Build history of the part. All positions in model axes, mm. Face numbers are marked on the shaded views. A direction names the side the tool comes from. Give positions to 0.01 mm unless a question says otherwise; leave off trailing zeros. Order: outer loops, then holes, each group sorted by start corner. A loop starts at its lowest first (then second) coordinate and runs counter-clockwise, first axis right, second up. Notation, with made-up numbers: (-14.5, 17.25) -> (34.5, 17.25) arc R10 ccw to (34.5, 28.25) -> close; hole circle Ø5 at (63, -24). An arc over 180 degrees is marked (long way). Write item = value, one per line. Start each with the question number.
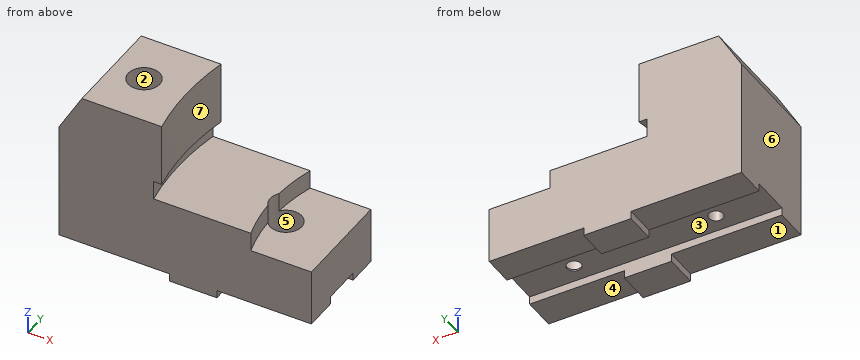
from build123d import *

# Parameters (mm, degrees)
SKETCH_W        = 160
SKETCH_H        = 65
PAD_DEPTH       = 100
POCKET_DEPTH    = 65.001
SKETCH002_R     = 4.5
POCKET001_DEPTH = 100.001
SKETCH003_R     = 10
POCKET002_DEPTH = 30
SKETCH004_R     = 170
POCKET003_DEPTH = 40
SKETCH005_R     = 175
POCKET004_DEPTH = 12
SKETCH006_R     = 115
POCKET005_DEPTH = 12
SKETCH007_R     = 4.5
POCKET006_DEPTH = 36.001
SKETCH008_R     = 10
POCKET009_DEPTH = 30
SKETCH009_W     = 30
SKETCH009_H     = 14.232688
PAD001_DEPTH    = 65
SKETCH010_W     = 25
SKETCH010_H     = 15.667085
POCKET010_DEPTH = 160.001


with BuildPart() as part:
    # Sketch → Pad (new body)
    with BuildSketch(Plane.XY):
        Rectangle(SKETCH_W, SKETCH_H)
    extrude(amount=PAD_DEPTH)

    # Sketch001 → Pocket (cut, through all)
    with BuildSketch(Plane.XZ.offset(32.5)):
        Polygon((-80, 100), (-80, 75), (-65.566243, 100), align=None)
    extrude(amount=-POCKET_DEPTH, mode=Mode.SUBTRACT)

    # Sketch002 → Pocket001 (cut, through all)
    with BuildSketch(Plane.XY.offset(100)):
        with Locations((-45, 0)):
            Circle(SKETCH002_R)
    extrude(amount=-POCKET001_DEPTH, mode=Mode.SUBTRACT)

    # Sketch003 → Pocket002 (cut)
    with BuildSketch(Plane.XY.offset(100)):
        with Locations((-45, 0)):
            Circle(SKETCH003_R)
    extrude(amount=-POCKET002_DEPTH, mode=Mode.SUBTRACT)

    # Sketch004 → Pocket003 (cut)
    with BuildSketch(Plane.XY.offset(100)):
        with Locations((151.864466, 0)):
            Circle(SKETCH004_R)
    extrude(amount=-POCKET003_DEPTH, mode=Mode.SUBTRACT)

    # Sketch005 → Pocket004 (cut)
    with BuildSketch(Plane.XY.offset(60)):
        with Locations((151.864466, 0)):
            Circle(SKETCH005_R)
    extrude(amount=-POCKET004_DEPTH, mode=Mode.SUBTRACT)

    # Sketch006 → Pocket005 (cut)
    with BuildSketch(Plane.XY.offset(48)):
        with Locations((151.864466, 0)):
            Circle(SKETCH006_R)
    extrude(amount=-POCKET005_DEPTH, mode=Mode.SUBTRACT)

    # Sketch007 → Pocket006 (cut, through all)
    with BuildSketch(Plane.XY.offset(36)):
        with Locations((45, 0)):
            Circle(SKETCH007_R)
    extrude(amount=-POCKET006_DEPTH, mode=Mode.SUBTRACT)

    # Sketch008 → Pocket009 (cut, symmetric)
    with BuildSketch(Plane.XY.offset(36)):
        with Locations((45, 0)):
            Circle(SKETCH008_R)
    extrude(amount=POCKET009_DEPTH, both=True, mode=Mode.SUBTRACT)

    # Sketch009 → Pad001 (new body)
    with BuildSketch(Plane.XZ.offset(32.5)):
        with Locations((5, 2.116344)):
            Rectangle(SKETCH009_W, SKETCH009_H)
    extrude(amount=-PAD001_DEPTH)

    # Sketch010 → Pocket010 (cut, through all)
    with BuildSketch(Plane.YZ.offset(80)):
        with Locations((0.638302, -2.833543)):
            Rectangle(SKETCH010_W, SKETCH010_H)
    extrude(amount=-POCKET010_DEPTH, mode=Mode.SUBTRACT)


solid = part.part
(1) Mould opens along X. For the marked faces 4, 5, 6 and 7 say: released by +X, released by -X, zero draft, split by the parting line, or undercut.
(2) Cut at C-C, the plane z = 16.5. Give the cut face in (x, y).
(3) Flat gauge pins, fed straight in: P1, Ø5.5, axis at y = 23, z = -3.5, coming from the -X side; P2, Ø10.5, axis at x = -49, y = -17.5, coming from the -Z side; P3, Ø10.5, axis at x = 45, y = 0, coming from the -Z side. Where does each tip first touch, or does it go through?
(4) Cut at A-A, the plane x = -45. Give the cut face in (y, z), plus the area to 3 significant figures.
(5) Cut at D-D, the plane x = 0. Give the cut face in (y, z), plus the area to 4 significant figures.
(6) 3-axis set-ups, long thin cutter, end or side, ignore diameter. For the marked faces 1, 2 and 3: which of +Z, -Z, +X, -X, +Y, -Y reach the whole face in a straight line?
(7) Cut at B-B, the plane y = 0. Give the cut face in (x, z).
(8) Wall check: line 1 (Y direction, x = 45, z = 16); line 2 (Y direction, x = 45, z = 5.85); line 3 (Z direction, x = 13.5, y = 19). Give the ranges that are in metal, low to high. Write a range as [from, to].
Results:
q1.face_4 = zero draft
q1.face_5 = undercut
q1.face_6 = released by -X
q1.face_7 = released by +X
q2.outline = (-80, -32.5) -> (80, -32.5) -> (80, 32.5) -> (-80, 32.5) -> close; hole circle Ø9 at (-45, 0); hole circle Ø20 at (45, 0)
q3.P1 = -10
q3.P2 = 0
q3.P3 = 5
q4.outline = (-32.5, 0) -> (-11.86, 0) -> (-11.86, 5) -> (-4.5, 5) -> (-4.5, 70) -> (-10, 70) -> (-10, 100) -> (-32.5, 100) -> close; (4.5, 5) -> (13.14, 5) -> (13.14, 0) -> (32.5, 0) -> (32.5, 100) -> (10, 100) -> (10, 70) -> (4.5, 70) -> close
q4.area = 5,190 mm2
q5.outline = (-32.5, -5) -> (-11.86, -5) -> (-11.86, 5) -> (13.14, 5) -> (13.14, -5) -> (32.5, -5) -> (32.5, 48) -> (-32.5, 48) -> close
q5.area = 3,195 mm2
q6.face_1 = -Z, -X, +Y, -Y
q6.face_2 = +Z
q6.face_3 = -Z, +X, -X
q7.outline = (-80, 5) -> (-49.5, 5) -> (-49.5, 70) -> (-55, 70) -> (-55, 100) -> (-65.57, 100) -> (-80, 75) -> close; (-40.5, 5) -> (40.5, 5) -> (40.5, 6) -> (35, 6) -> (35, 48) -> (-23.14, 48) -> (-23.14, 60) -> (-18.14, 60) -> (-18.14, 100) -> (-35, 100) -> (-35, 70) -> (-40.5, 70) -> close; (49.5, 5) -> (80, 5) -> (80, 36) -> (55, 36) -> (55, 6) -> (49.5, 6) -> close
q8.line_1 = [-32.5, -10], [10, 32.5]
q8.line_2 = [-32.5, -4.5], [4.5, 32.5]
q8.line_3 = [-5, 48]
